Read the model definition and answer for the solid it produces. Units are mm, in the model's axes. A direction names the side the tool comes from. Give positions to 0.01 mm unless a question says otherwise; leave off trailing zeros. Loops run counter-clockwise (first coordinate to the right, second up) from the corner with the lowest first, then second, coordinate; pieces in that order, holes last. Notation, with made-up numbers: (-22.75, 73) - (-3.75, 73) arc R22 ccw to (-3.75, 106) - close; hole circle Ø2 at (32.5, 84.25). An arc over 180 degrees is marked (long way). Put each result on its own line as item: value. Start each with the question number.
1. For faces 1 (the flat face through (-4, -9, -4)), 2 (the flat face through (5, -7, -10)), 3 (the flat face through (-1.5, 0, -6)), determine the directions among +Z, -Z, +X, -X, +Y, -Y from which every point of the face is accessible in a straight line to the end or side of a thin tool.
2. A cutting plane is placed at A-A, the plane y = 6. Determine the outline of the cut face in (x, z).
3. Given pin 1 Ø1.5 at (x, z) = (6.5, 8.5) entering from -Y; pin 2 Ø5 at (x, z) = (11, -12) entering from +Y; pin 3 Ø1.3 at (y, z) = (4.5, -5.5) entering from -X, each flat-ended and moving along its own axis, determine where each tip first touches the part or whether it passes through.
4. Consider L1, parallel to Z at x = 0, y = 3; L2, parallel to X at y = 2.5, z = 0; L3, parallel to Z at x = -3, y = 1. Determine where each line is inside the solid, lowest interval first. Write a range as from..to.
5. A cutting plane is placed at B-B, the plane y = -1. Determine the outline of the cut face in (x, z), plus the area to 3 significant figures.
6. For a pull along X with two mould halves and no side action, classify faces 4 (the cylindrical face through (0, 0, 5)), 5 (the flat face through (-4, 9, 4)), 6 (the conical face through (-8.753, 8.875, 1.944)) as released by +X, released by -X, zero draft, split by the parting line, or undercut.
```python
from build123d import *

# Parameters (mm, degrees)
SKETCH_2_W          = 3
SKETCH_2_H          = 2.405661247
CUT_EXTRUDE_1_DEPTH = 19


with BuildPart() as part:
    # Эскиз1 → Повернуть1 (revolve)
    with BuildSketch(Plane(origin=(0, 0, 0), x_dir=(0, 0, -1), z_dir=(1, 0, 0))):
        with BuildLine():
            Line((15, 7), (15, 5))
            ThreePointArc((15, 5), (14.5, 4.5), (15, 4))
            Line((15, 4), (14.982695469, -3.900561726))
            ThreePointArc((14.982695469, -3.900561726), (14.409213991, -4.525956797), (15.034609063, -5.099438274))
            Line((15.034609063, -5.099438274), (15.034609063, -7))
            Line((15.034609063, -7), (10.850882415, -7))
            Line((10.850882415, -7), (8.840023423, -9))
            Line((8.840023423, -9), (5, -9))
            Line((5, -9), (5, 9))
            Line((5, 9), (8.840023423, 9))
            Line((8.840023423, 9), (10.850882415, 7))
            Line((10.850882415, 7), (15, 7))
        make_face()
    revolve(axis=Axis((0, 26.633173064, 0), (0, -1, 0)))

    # Эскиз2 → Вырез-Вытянуть1 (cut, through all)
    with BuildSketch(Plane(origin=(0, 9, 0), x_dir=(1, 0, 0), z_dir=(0, 1, 0))):
        with Locations((0, 5.202830624)):
            Rectangle(SKETCH_2_W, SKETCH_2_H)
    extrude(amount=-CUT_EXTRUDE_1_DEPTH, mode=Mode.SUBTRACT)


solid = part.part
```
Return value:
1. face 1: +Z, -Z, +X, -X, -Y
1. face 2: -Y
1. face 3: +Y, -Y
2. outline: circle Ø30 at (0, 0); hole (-1.5, -6.41) - (1.5, -6.41) - (1.5, -4.77) arc R5 ccw (long way) to (-1.5, -4.77) - close
3. pin 1: stops at y = -7.9
3. pin 2: stops at y = 7
3. pin 3: stops at x = -14.11
4. L1: z = -15..-6.41, 5..15
4. L2: x = -15..-5, 5..15
4. L3: z = -14.69..-4, 4..14.69
5. outline: circle Ø29.98 at (0, 0); hole (-1.5, -6.41) - (1.5, -6.41) - (1.5, -4.77) arc R5 ccw (long way) to (-1.5, -4.77) - close
5. area: 623 mm2
6. face 4: undercut
6. face 5: zero draft
6. face 6: split by the parting line
